Verification items for the finished model (mm, model axes). Face numbers are marked on the shaded views. A direction names the side the tool comes from. Coordinates: 2 decimals unless noted, no trailing zeros. Order: outer loops, then holes, each group sorted by start corner. A loop starts at its lowest first (then second) coordinate and runs counter-clockwise, first axis right, second up.
Q1. Depth check by flat-ended pin: P1, Ø4, axis at x = 0, z = 0, coming from the -Y side; P2, Ø1.8, axis at y = 1.5, z = -7.5, coming from the +X side; P3, Ø1.1, axis at x = 0, y = 1.5, coming from the -Z side; P4, Ø2, axis at x = 7.5, y = 2, coming from the -Z side. Enter the tip coordinate at first touch or a pass-through.
Q2. Thickness scan on line 1 (X direction, y = 3.85, z = 0); line 2 (X direction, y = 1.15, z = 3.5); line 3 (X direction, y = 2.45, z = -5.5). Record the ranges inside material, lowest first.
Q3. Draft check along Z on the marked faces 4, 5, 6 and 7. Enter one of: pulls with the +Z half, pulls with the -Z half, needs draft (parallel to the pull), parting line crosses it, or undercut.
Q4. Cross-section at B-B, the plane x = 0. Record the boundary of the cut face in (y, z).
Q5. Cross-section at D-D, the plane y = 2.25. Record the boundary of the cut face in (x, z), and give its area (3 significant figures).
Q6. Cross-section at C-C, the plane z = 0. Record the boundary of the cut face in (x, y), and give its area (3 significant figures).
Q7. Set-up check for the marked faces 1, 2 and 3: record each of +Z, -Z, +X, -X, +Y, -Y from which the full face is reachable in a straight line by a thin tool's end or side.
Q8. Cross-section at A-A, the plane z = 2. Record the boundary of the cut face in (x, y).
from build123d import *

# Parameters (mm, degrees)
SKETCH_1_W          = 20
SKETCH_1_H          = 20
EXTRUDE_1_DEPTH     = 5
SKETCH_2_R          = 2.55
CUT_EXTRUDE_1_DEPTH = 5
SKETCH_3_W          = 5
SKETCH_3_H          = 6.1
CUT_EXTRUDE_2_DEPTH = 5
SKETCH_5_R          = 1
CUT_EXTRUDE_4_DEPTH = 10
FILLET_1_R          = 5
SKETCH_6_W          = 6
SKETCH_6_H          = 5
CUT_EXTRUDE_5_DEPTH = 10
SKETCH_7_R          = 1
CUT_EXTRUDE_6_DEPTH = 10
SKETCH_8_R          = 1.25
CUT_EXTRUDE_7_DEPTH = 5


with BuildPart() as part:
    # 스케치1 → 보스-돌출1 (new body)
    with BuildSketch(Plane(origin=(0, 0, 0), x_dir=(1, 0, 0), z_dir=(0, 1, 0))):
        Rectangle(SKETCH_1_W, SKETCH_1_H)
    extrude(amount=EXTRUDE_1_DEPTH)

    # 스케치2 → 컷-돌출1 (cut)
    with BuildSketch(Plane(origin=(0, 5, 0), x_dir=(1, 0, 0), z_dir=(0, 1, 0))):
        with Locations(Location((0, 0, 0), (0, 0, 270))):
            Circle(SKETCH_2_R)
    extrude(amount=-CUT_EXTRUDE_1_DEPTH, mode=Mode.SUBTRACT)

    # 스케치3 → 컷-돌출2 (cut)
    with BuildSketch(Plane.XZ):
        with Locations((0, 3.05)):
            Rectangle(SKETCH_3_W, SKETCH_3_H)
    extrude(amount=-CUT_EXTRUDE_2_DEPTH, mode=Mode.SUBTRACT)

    # 스케치5 → 컷-돌출4 (cut)
    with BuildSketch(Plane(origin=(0, 0, 0), x_dir=(-1, 0, 0), z_dir=(0, -1, 0))):
        with Locations((-1.792893219, -5.392893219)):
            Circle(SKETCH_5_R)
        with Locations((1.792893219, -5.392893219)):
            Circle(SKETCH_5_R)
    extrude(amount=-CUT_EXTRUDE_4_DEPTH, mode=Mode.SUBTRACT)

    # 필렛1
    fillet_1_edges = [part.edges().sort_by_distance(p)[0] for p in [
        (10, 2.5, 10),
        (-10, 2.5, 10),
        (-10, 2.5, -10),
        (10, 2.5, -10),
    ]]
    fillet(fillet_1_edges, radius=FILLET_1_R)

    # 스케치6 → 컷-돌출5 (cut)
    with BuildSketch(Plane.XZ):
        with Locations((0, -7.5)):
            Rectangle(SKETCH_6_W, SKETCH_6_H)
    extrude(amount=-CUT_EXTRUDE_5_DEPTH, mode=Mode.SUBTRACT)

    # 스케치7 → 컷-돌출6 (cut)
    with BuildSketch(Plane(origin=(0, 0, 0), x_dir=(-1, 0, 0), z_dir=(0, -1, 0))):
        with Locations((-2.292893219, 5.707106781)):
            Circle(SKETCH_7_R)
        with Locations((2.292893219, 5.707106781)):
            Circle(SKETCH_7_R)
    extrude(amount=-CUT_EXTRUDE_6_DEPTH, mode=Mode.SUBTRACT)

    # 스케치8 → 컷-돌출7 (cut)
    with BuildSketch(Plane.XZ):
        with Locations(Location((4.949747468, 4.949747468, 0), (0, 0, 270))):
            Circle(SKETCH_8_R)
        with Locations(Location((7, 0, 0), (0, 0, 270))):
            Circle(SKETCH_8_R)
        with Locations(Location((4.949747468, -4.949747468, 0), (0, 0, 270))):
            Circle(SKETCH_8_R)
        with Locations(Location((-4.949747468, -4.949747468, 0), (0, 0, 270))):
            Circle(SKETCH_8_R)
        with Locations(Location((-7, 0, 0), (0, 0, 270))):
            Circle(SKETCH_8_R)
        with Locations(Location((-4.949747468, 4.949747468, 0), (0, 0, 270))):
            Circle(SKETCH_8_R)
    extrude(amount=-CUT_EXTRUDE_7_DEPTH, mode=Mode.SUBTRACT)


solid = part.part
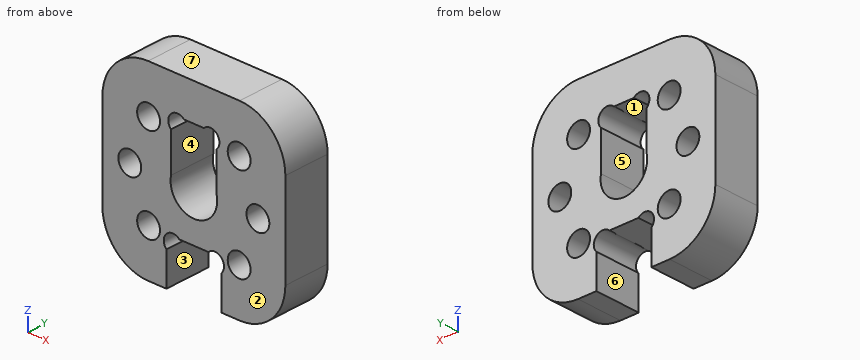
Check values:
1. P1: passes through
1. P2: stops at x = 9.74
1. P3: stops at z = -5
1. P4: stops at z = -9.77
2. line 1: x = -10 to -8.25, -5.75 to -2.55, 2.55 to 5.75, 8.25 to 10
2. line 2: x = -10 to -2.5, 2.5 to 10
2. line 3: x = -9.97 to -6.07, -3.83 to -3.27, 3.27 to 3.83, 6.07 to 9.97
3. face 4: undercut
3. face 5: undercut
3. face 6: needs draft
3. face 7: pulls with the +Z half
4. outline: (0, -5) - (5, -5) - (5, -2.55) - (0, -2.55) - close; (0, 6.1) - (5, 6.1) - (5, 10) - (0, 10) - close
5. outline: (-10, -5) arc R5 ccw to (-5, -10) - (-3, -10) - (-3, -6.41) arc R1 cw to (-1.59, -5) - (1.59, -5) arc R1 cw to (3, -6.41) - (3, -10) - (5, -10) arc R5 ccw to (10, -5) - (10, 5) arc R5 ccw to (5, 10) - (-5, 10) arc R5 ccw to (-10, 5) - close; hole circle Ø2.5 at (-7, 0); hole circle Ø2.5 at (-4.95, -4.95); hole circle Ø2.5 at (-4.95, 4.95); hole (-2.5, 0.5) arc R2.55 ccw (long way) to (2.5, 0.5) - (2.5, 4.69) arc R1 ccw to (1.09, 6.1) - (-1.09, 6.1) arc R1 ccw to (-2.5, 4.69) - close; hole circle Ø2.5 at (4.95, -4.95); hole circle Ø2.5 at (4.95, 4.95); hole circle Ø2.5 at (7, 0)
5. area: 276 mm2
6. outline: (-10, 0) - (-8.25, 0) - (-8.25, 5) - (-10, 5) - close; (-5.75, 0) - (-2.55, 0) - (-2.55, 5) - (-5.75, 5) - close; (2.55, 0) - (5.75, 0) - (5.75, 5) - (2.55, 5) - close; (8.25, 0) - (10, 0) - (10, 5) - (8.25, 5) - close
6. area: 49.5 mm2
7. face 1: +Y, -Y
7. face 2: +Z, -Z, +X, -X, -Y
7. face 3: -Z, +Y, -Y
8. outline: (-10, 0) - (-2.5, 0) - (-2.5, 5) - (-10, 5) - close; (2.5, 0) - (10, 0) - (10, 5) - (2.5, 5) - close
